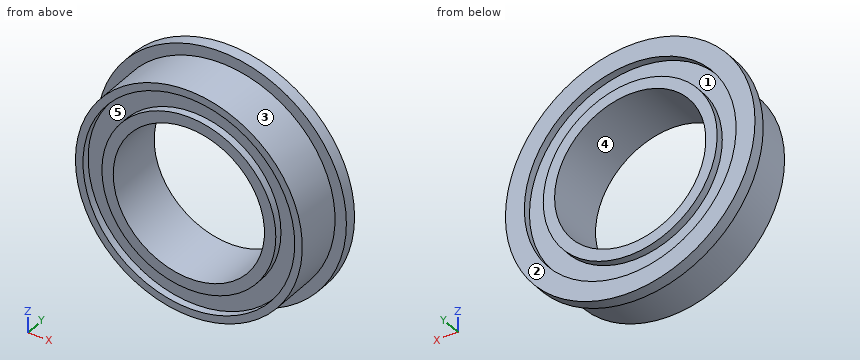
Autodesk Inventor part; units mm, degrees
ref_plane "YZ Plane" through (0, 0, 0) normal (1, 0, 0) x (0, 1, 0)
ref_plane "XZ Plane" through (0, 0, 0) normal (0, 1, 0) x (-1, 0, 0)
ref_plane "XY Plane" through (0, 0, 0) normal (0, 0, 1) x (1, 0, 0)
sketch "Sketch1" plane through (0, 0, 0) normal (0, 1, 0) x (-1, 0, 0)
  circle A0 centre (0, 0) radius 5
  circle A1 centre (0, 0) radius 7.5
  dimension "d0" = 10
  dimension "d1" = 15
extrude "Extrusion1" add sketch "Sketch1" along normal blind 3.2
sketch "Sketch2" plane through (0, 3.2, 0) normal (0, 1, 0) x (1, 0, 0)
  circle A0 centre (0, 0) radius 5
  circle A1 centre (0, 0) radius 8.25
  dimension "d4" = 16.5
extrude "Extrusion2" add sketch "Sketch2" along normal blind 0.8
sketch "Sketch3" plane through (0, 4, 0) normal (0, 1, 0) x (1, 0, 0)
  circle A0 centre (0, 0) radius 5.75
  circle A1 centre (0, 0) radius 7
  dimension "d7" = 11.5
  dimension "d8" = 14
extrude "Extrusion3" cut sketch "Sketch3" against normal blind 0.5
sketch "Sketch4" plane through (0, 0, 0) normal (0, -1, 0) x (1, 0, 0)
  circle A0 centre (0, 0) radius 7
  circle A1 centre (0, 0) radius 5.75
extrude "Extrusion4" cut sketch "Sketch4" against normal blind 0.5
properties part number "10x15x4mm Flanged Bearing"
Check sheet for the modelled part. Datum: model origin and axes. Units: mm. Face numbers are marked on the shaded views. A direction names the side the tool comes from. Round coordinates to 2 decimals unless told otherwise and drop trailing zeros. Loops run counter-clockwise (first coordinate to the right, second up) from the corner with the lowest first, then second, coordinate; pieces in that order, holes last. Notation, with made-up numbers: (11.25, -16) -> (35.25, -16) arc R12 cw to (35.25, -9) -> close; hole circle Ø10 at (-28, 75.5). An arc over 180 degrees is marked (long way). Answer in a Markdown table with one row per item.
Q1. Sectioned sample at A-A on z = -4.25. Enter the section's corners in (x, y).
Data:
| item | result |
|---|---|
| outline | (-7.07, 3.2) -> (-6.18, 3.2) -> (-6.18, 0) -> (-5.56, 0) -> (-5.56, 0.5) -> (-3.87, 0.5) -> (-3.87, 0) -> (-2.63, 0) -> (-2.63, 4) -> (-3.87, 4) -> (-3.87, 3.5) -> (-5.56, 3.5) -> (-5.56, 4) -> (-7.07, 4) -> close; (2.63, 0) -> (3.87, 0) -> (3.87, 0.5) -> (5.56, 0.5) -> (5.56, 0) -> (6.18, 0) -> (6.18, 3.2) -> (7.07, 3.2) -> (7.07, 4) -> (5.56, 4) -> (5.56, 3.5) -> (3.87, 3.5) -> (3.87, 4) -> (2.63, 4) -> close |
Q2. Release check for a two-part mould opening along X. For the marked faces 1, 2 and 3 record: released by +X, released by -X, zero draft, split by the parting line, or undercut.
Data:
| item | result |
|---|---|
| face 1 | undercut |
| face 2 | zero draft |
| face 3 | split by the parting line |
Q3. Set-up check for the marked faces 4 and 5: record each of +Z, -Z, +X, -X, +Y, -Y from which the full face is reachable in a straight line by a thin tool's end or side.
Data:
| item | result |
|---|---|
| face 4 | +Y, -Y |
| face 5 | -Y |
Q4. Sectioned sample at C-C on y = 2.95. Enter the section's corners in (x, z), then the cut area to 3 significant figures.
Data:
| item | result |
|---|---|
| outline | circle Ø15 at (0, 0); hole circle Ø10 at (0, 0) |
| area | 98.2 mm^2 |
Q5. Thickness scan on L1, parallel to X at y = 3.75, z = 0; L2, parallel to X at y = 3.8, z = 1.25. Record the ranges inside material, lowest first.
Data:
| item | result |
|---|---|
| L1 | x = -8.25 to -7, -5.75 to -5, 5 to 5.75, 7 to 8.25 |
| L2 | x = -8.15 to -6.89, -5.61 to -4.84, 4.84 to 5.61, 6.89 to 8.15 |
Q6. Go/stop test with flat-tipped pins: P1, Ø7, axis at x = 1, z = -2.5, coming from the +Y side; P2, Ø1.5, axis at y = 3.5, z = 5.5, coming from the -X side. Record where each tip stops, or that it passes through.
Data:
| item | result |
|---|---|
| P1 | stops at y = 4 |
| P2 | stops at x = -6.75 |
